For this review, take the finished solid that the model builds, in its own axes (mm). Face numbers are marked on the shaded views. A direction names the side the tool comes from. Round coordinates to 2 decimals unless told otherwise and drop trailing zeros. Write each loop counter-clockwise with the first axis right and the second up, starting at its lowest first coordinate (ties: lowest second). Pieces come first, ordered by that corner, then holes. Notation, with made-up numbers: (-21.5, 72) - (4.5, 72) arc R25 ccw to (4.5, 88) - close; hole circle Ø8 at (35.25, -6.75). An arc over 180 degrees is marked (long way). Answer in a Markdown table with one row per item. Add a question column.
from build123d import *

# Parameters (mm, degrees)
SKETCH170_R     = 1.55
PAD089_DEPTH    = 2.5
PAD090_DEPTH    = 11
SKETCH172_R     = 1.5
POCKET066_DEPTH = 5
SKETCH_R        = 1.75
POCKET_DEPTH    = 5
CHAMFER_SIZE    = 1


with BuildPart() as part:
    # Sketch170 → Pad089 (new body)
    with BuildSketch(Plane.YZ):
        with BuildLine():
            ThreePointArc((-10.7502555542, 27.7356075645), (-14.2856053806, 27.6997466745), (-14.2497489032, 24.1643968034))
            Line((-14.2497489032, 24.1643968034), (-10, 20))
            Line((-10, 20), (-10, 0))
            Line((-10, -20), (-10, 0))
            Line((-14.2497550835, -24.1644028597), (-10, -20))
            ThreePointArc((-14.2497550835, -24.1644028597), (-14.2855992835, -27.6997528965), (-10.7502492905, -27.7356014266))
            Line((-10.7502492905, -27.7356014266), (-6.5005101735, -23.5712142128))
            Line((-6.5005101735, -23.5712142128), (6.5005101735, -23.5712142128))
            Line((10.7502488005, -27.7356009464), (6.5005101735, -23.5712142128))
            ThreePointArc((10.7502488005, -27.7356009464), (14.2856010292, -27.699751115), (14.2497510305, -24.164398888))
            Line((14.2497510305, -24.164398888), (10, -20))
            Line((10, -20), (10, 0))
            Line((10, 20), (10, 0))
            Line((14.2497448501, 24.1643928317), (10, 20))
            ThreePointArc((14.2497448501, 24.1643928317), (14.2856070566, 27.6997449641), (10.7502549219, 27.7356069449))
            Line((10.7502549219, 27.7356069449), (6.5005101735, 23.5712142128))
            Line((6.5005101735, 23.5712142128), (0, 23.5712142128))
            Line((-6.5005101735, 23.5712142128), (0, 23.5712142128))
            Line((-10.7502555542, 27.7356075645), (-6.5005101735, 23.5712142128))
        make_face()
        with Locations((-12.5, 25.95)):
            Circle(SKETCH170_R, mode=Mode.SUBTRACT)
        with Locations((12.5, 25.95)):
            Circle(SKETCH170_R, mode=Mode.SUBTRACT)
        with Locations((-12.5, -25.95)):
            Circle(SKETCH170_R, mode=Mode.SUBTRACT)
        with Locations((12.5, -25.95)):
            Circle(SKETCH170_R, mode=Mode.SUBTRACT)
    extrude(amount=PAD089_DEPTH)

    # Sketch171 (on DatumPlane) → Pad090 (join, symmetric)
    with BuildSketch(Plane(origin=(2.5, 0, 0), x_dir=(0, 1, 0), z_dir=(0, 0, -1))):
        Polygon((-13.4350288425, 17.1213203436), (-14.8492424049, 15.7071067812), (-3.5, 4.3578643763), (-3.5, 0), (3.5, 0), (3.5, 10.0147186258), (12.0208152802, 18.5355339059), (10.6066017178, 19.9497474683), (2.8284271247, 12.1715728753), (0, 15), (-5.6568542495, 9.3431457505), align=None)
    extrude(amount=PAD090_DEPTH, both=True)

    # Sketch172 (on Face30 of Pad090) → Pocket066 (cut)
    with BuildSketch(Plane(origin=(1.6789321881, 1.6789321881, 0), x_dir=(-0.7071067812, 0.7071067812, 0), z_dir=(-0.7071067812, -0.7071067812, 0))):
        with Locations((-19.8743686708, -6.5)):
            Circle(SKETCH172_R)
        with BuildLine():
            ThreePointArc((-22.7830913882, -4.5533792991), (-22.9517672177, -8.1672186969), (-19.8324532872, -9.9997490054))
            Line((-19.8324532872, -9.9997490054), (-12.3743686708, -11))
            Line((-12.3743686708, -11), (-12.3743686708, -12))
            Line((-12.3743686708, -12), (-25.675823, -12))
            Line((-25.675823, -12), (-25.675823, 11.874653))
            Line((-25.675823, 11.874653), (-12.3743686708, 11.874653))
            Line((-12.3743686708, 11.874653), (-12.3743686708, 11))
            Line((-12.3743686708, 11), (-22.7830913882, -4.5533792991))
        make_face()
    extrude(amount=-POCKET066_DEPTH, mode=Mode.SUBTRACT)

    # Sketch (on Face33 of Pocket066) → Pocket (cut)
    with BuildSketch(Plane(origin=(5.9215728753, -5.9215728753, 0), x_dir=(0, 0, -1), z_dir=(0.7071067812, -0.7071067812, 0))):
        with Locations((6.5, 19.8743686708)):
            Circle(SKETCH_R)
        with BuildLine():
            Line((9.9710425685, 20.3236608785), (11, 12.3743686708))
            Line((11, 12.3743686708), (13.188866, 12.3743686708))
            Line((13.188866, 12.3743686708), (13.237601, 26.90383))
            Line((13.237601, 26.90383), (-12.122474, 26.90383))
            Line((-12.122474, 26.90383), (-12.122474, 12.372268))
            Line((-12.122474, 12.372268), (-11, 12.3743686708))
            Line((-11, 12.3743686708), (4.5533989217, 22.7831045202))
            ThreePointArc((9.9710425685, 20.3236608785), (7.9467882433, 23.0613427496), (4.5533989217, 22.7831045202))
        make_face()
    extrude(amount=-POCKET_DEPTH, mode=Mode.SUBTRACT)

    # Chamfer
    chamfer_edges = [part.edges().sort_by_distance(p)[0] for p in [
        (2.5, 0, -11),
        (2.5, 3.5, 0),
        (2.5, -3.5, 0),
        (2.5, 0, 11),
        (6.857864, -3.5, 0),
        (12.514719, 3.5, 0),
        (17.5, 0, 0),
    ]]
    chamfer(chamfer_edges, length=CHAMFER_SIZE)


solid = part.part
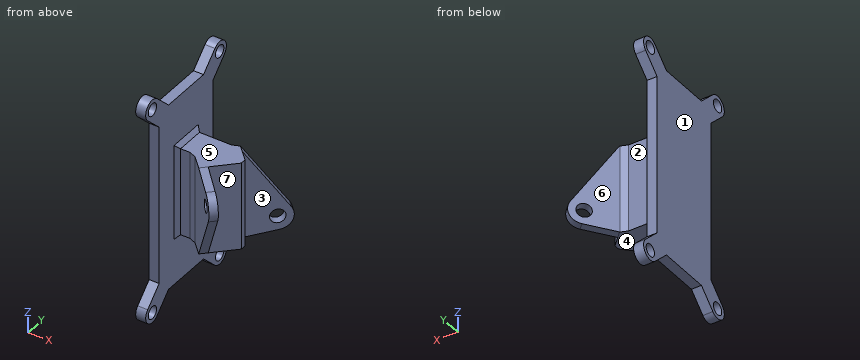
Q1. Draft analysis for pull direction Y (two halves, no side actions). For the marked faces 5, 6 and 7, state which applies: released by +Y, released by -Y, zero draft, split by the parting line, or undercut.
Q2. Tool access review of the marked faces 1, 2, 3 and 4: name each direction out of +Z, -Z, +X, -X, +Y, -Y from which nothing blocks a thin tool from reaching the whole face with its end or side.
Q3. To check wall thickness, follow probe 1 along Z at (x, y) = (0.7, -12.5); probe 2 along Z at (x, y) = (2, -12); probe 3 along Y at (x, z) = (15.25, 6). State the ranges of each line that lie inside material, in increasing order.
Q4. Add section B-B on z = -15. State the section outline as (x, y) points.
Q5. Add section C-C on z = -22. State the section outline as (x, y) points, then the cut area to 3 significant figures.
Q6. Insertion check: pin 1 Ø6 at (x, y) = (9.5, -9.5) entering from +Z; pin 2 Ø12.5 at (x, y) = (12, -2.5) entering from -Z; pin 3 Ø0.7 at (x, z) = (4, -4.5) entering from -Y. Each pin has a flat end and moves straight along its axis. Give the tip position at first contact, or say it passes through.
Q7. Add section A-A on z = 25.95. State the section outline as (x, y) points.
Answer sheet:
| question | item | result |
|---|---|---|
| 1 | face 5 | zero draft |
| 1 | face 6 | released by +Y |
| 1 | face 7 | undercut |
| 2 | face 1 | +Z, -Z, -X, +Y, -Y |
| 2 | face 2 | +Z, -Z, +Y |
| 2 | face 3 | +Z, -Z, +X |
| 2 | face 4 | -Z, +X, +Y, -Y |
| 3 | probe 1 | z = -28.45 to -27.5, -24.4 to -22.45, 22.45 to 24.4, 27.5 to 28.45 |
| 3 | probe 2 | z = -28.4 to -27.42, -24.48 to -21.96, 21.96 to 24.48, 27.42 to 28.4 |
| 3 | probe 3 | y = -10.86 to -9.06, -2.25 to 2.25, 3.41 to 6.24 |
| 4 | outline | (0, -10) - (2.5, -10) - (2.5, 10) - (0, 10) - close |
| 5 | outline | (0, -12.04) - (2.5, -12.04) - (2.5, 12.04) - (0, 12.04) - close |
| 5 | area | 60.2 mm² |
| 6 | pin 1 | stops at z = 11 |
| 6 | pin 2 | stops at z = -11 |
| 6 | pin 3 | stops at y = -3.5 |
| 7 | outline | (0, -15) - (2.5, -15) - (2.5, -14.05) - (0, -14.05) - close; (0, -10.95) - (2.5, -10.95) - (2.5, -8.93) - (0, -8.93) - close; (0, 8.93) - (2.5, 8.93) - (2.5, 10.95) - (0, 10.95) - close; (0, 14.05) - (2.5, 14.05) - (2.5, 15) - (0, 15) - close |
